```python
from build123d import *

# Parameters (mm, degrees)
F0_W      = 100
F0_H      = 115
F1_DEPTH  = 15
F2_R      = 23
F3_DEPTH  = 4
F5_R      = 4.7
F6_DEPTH  = 91
F7_R      = 8
F8_DEPTH  = 7
F9_R      = 4.25
F10_DEPTH = 82
F11_W     = 27
F11_H     = 8
F12_DEPTH = 7.5
F14_DEPTH = 20
F15_DEPTH = 4
F16_R     = 5
F17_DEPTH = 4


with BuildPart() as f1:
    # F0 (on Top) → F1 (new body)
    with BuildSketch(Plane.XY):
        with Locations((50, 57.5)):
            Rectangle(F0_W, F0_H)
    extrude(amount=F1_DEPTH)

    # F2 (on face) → F3 (cut)
    with BuildSketch(Plane.XY.offset(15)):
        with Locations((70, 85)):
            Circle(F2_R)
    extrude(amount=-F3_DEPTH, mode=Mode.SUBTRACT)

    # F5 (on offset) → F6 (cut)
    with BuildSketch(Plane(origin=(0, 108, 0), x_dir=(-1, 0, 0), z_dir=(0, 1, 0))):
        with Locations((-14.4, 14)):
            Circle(F5_R)
    extrude(amount=-F6_DEPTH, mode=Mode.SUBTRACT)

    # F7 (on face) → F8 (cut)
    with BuildSketch(Plane(origin=(0, 17, 0), x_dir=(-1, 0, 0), z_dir=(0, 1, 0))):
        with Locations((-14.4, 14)):
            Circle(F7_R)
        with BuildLine():
            ThreePointArc((-9.8076149987, 15), (-14.4, 9.3), (-18.9923850013, 15))
            Line((-18.9923850013, 15), (-9.8076149987, 15))
        make_face(mode=Mode.SUBTRACT)
        with BuildLine():
            Line((-9.8076149987, 15), (-18.9923850013, 15))
            ThreePointArc((-18.9923850013, 15), (-14.4, 9.3), (-9.8076149987, 15))
        make_face()
    extrude(amount=-F8_DEPTH, mode=Mode.SUBTRACT)

    # F9 (on offset) → F10 (cut)
    with BuildSketch(Plane(origin=(0, 108, 0), x_dir=(-1, 0, 0), z_dir=(0, 1, 0))):
        with Locations((-34.4, 14)):
            Circle(F9_R)
    extrude(amount=-F10_DEPTH, mode=Mode.SUBTRACT)

    # F11 (on face) → F12 (cut)
    with BuildSketch(Plane.XY.offset(15)):
        with Locations((70, 48)):
            Rectangle(F11_W, F11_H)
    extrude(amount=-F12_DEPTH, mode=Mode.SUBTRACT)

    # F13 (on face) → F14 (cut)
    with BuildSketch(Plane(origin=(0, 44, 0), x_dir=(-1, 0, 0), z_dir=(0, 1, 0))):
        Polygon((-79.75, 14.9995335633), (-79.75, 12.719), (-77.775, 11.5787332184), (-75.8, 12.719), (-75.8, 14.9995335633), (-75.8008078921, 15), (-79.7491921079, 15), align=None)
        Polygon((-68.0508078921, 15), (-71.9991921079, 15), (-72, 14.9995335633), (-72, 12.719), (-70.025, 11.5787332184), (-68.05, 12.719), (-68.05, 14.9995335633), align=None)
        Polygon((-60.3008078921, 15), (-64.2491921079, 15), (-64.25, 14.9995335633), (-64.25, 12.719), (-62.275, 11.5787332184), (-60.3, 12.719), (-60.3, 14.9995335633), align=None)
    extrude(amount=-F14_DEPTH, mode=Mode.SUBTRACT)

    # F15 (cut): a face of the model
    f15_faces = [f1.faces().sort_by_distance(p)[0] for p in [
        (70, 52, 11.25),
    ]]
    extrude(f15_faces, amount=-F15_DEPTH, mode=Mode.SUBTRACT)

    # F16
    f16_edges = [f1.edges().sort_by_distance(p)[0] for p in [
        (50, 0, 15),
        (100, 57.5, 15),
        (50, 115, 15),
        (0, 57.5, 15),
        (100, 115, 7.5),
        (0, 115, 7.5),
        (100, 0, 7.5),
        (0, 0, 7.5),
        (56.5, 50, 7.5),
        (83.5, 50, 7.5),
    ]]
    fillet(f16_edges, radius=F16_R)

    # F17 (cut): a face of the model
    f17_faces = [f1.faces().sort_by_distance(p)[0] for p in [
        (50, 57.5, 0),
    ]]
    extrude(f17_faces, amount=-F17_DEPTH, mode=Mode.SUBTRACT)


solid = f1.part
```
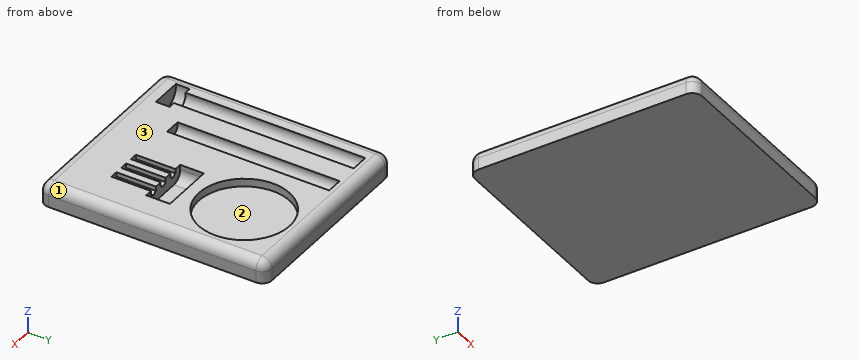
For this review, take the finished solid that the model builds, in its own axes (mm). Face numbers are marked on the shaded views. Round coordinates to 2 decimals unless told otherwise and drop trailing zeros. Write each loop counter-clockwise with the first axis right and the second up, starting at its lowest first coordinate (ties: lowest second). Pieces come first, ordered by that corner, then holes. Notation, with made-up numbers: (25.25, 48.25) - (49.25, 48.25) arc R18 cw to (49.25, 83.25) - close; hole circle Ø7 at (3, -23). An arc over 180 degrees is marked (long way). Answer as a JSON object with one key per item and string values.
1. To check wall thickness, follow line 1 along Y through (x, z) = (69, 12); line 2 along X through (y, z) = (58, 11.5); line 3 along Y through (x, z) = (16, 7.5). State the ranges of each line that lie inside material, in increasing order.
Response values:
{"line 1": "y = 0.42 to 44, 56 to 62.02, 107.98 to 114.58", "line 2": "x = 0.23 to 10.42, 18.38 to 30.96, 37.84 to 99.77", "line 3": "y = 0 to 10, 17 to 115"}
2. We need section B-B on y = 65. Give the boundary of the cut face in (x, z), then the cut area to 3 significant figures.
Response values:
{"outline": "(0, 4) - (100, 4) - (100, 10) arc R5 ccw to (95, 15) - (81.36, 15) - (81.36, 11) - (58.64, 11) - (58.64, 15) - (38.53, 15) arc R4.25 cw (long way) to (30.27, 15) - (18.99, 15) arc R4.7 cw (long way) to (9.81, 15) - (5, 15) arc R5 ccw to (0, 10) - close", "area": "918 mm2"}
3. Draft analysis for pull direction X (two halves, no side actions). For the marked faces 1, 2 and 3, state which applies: +X half, -X half, draft (parallel to the pull), parting line (faces both ways), or undercut.
Response values:
{"face 1": "+X half", "face 2": "undercut", "face 3": "draft"}
4. We need section C-C on x = 89. Give the boundary of the cut face in (y, z), then the cut area to 3 significant figures.
Response values:
{"outline": "(0, 4) - (115, 4) - (115, 10) arc R5 ccw to (110, 15) - (97.96, 15) - (97.96, 11) - (72.04, 11) - (72.04, 15) - (5, 15) arc R5 ccw to (0, 10) - close", "area": "1,150 mm2"}
5. For pin 1 Ø0.8 at (y, z) = (51.5, 13) entering from +X; pin 2 Ø1.7 at (x, z) = (78, 13.5) entering from +Y; pin 3 Ø9.5 at (x, y) = (70, 50) entering from +Z, all flat-tipped, find the tip position at first contact; note any pin that passes through.
Response values:
{"pin 1": "stops at x = 99.27", "pin 2": "stops at y = 114.24", "pin 3": "stops at z = 7.5"}
6. We need section A-A on x = 14.4. Give the boundary of the cut face in (y, z), then the cut area to 3 significant figures.
Response values:
{"outline": "(0, 4) - (115, 4) - (115, 10) arc R5 ccw to (110, 15) - (108, 15) - (108, 9.3) - (17, 9.3) - (17, 6) - (10, 6) - (10, 15) - (5, 15) arc R5 ccw to (0, 10) - close", "area": "673 mm2"}
